Build history of the part. All positions in model axes, mm. Round coordinates to 2 decimals unless told otherwise and drop trailing zeros. Loops run counter-clockwise (first coordinate to the right, second up) from the corner with the lowest first, then second, coordinate; pieces in that order, holes last. Notation, with made-up numbers: (22, 79.5) - (56, 79.5) arc R25 cw to (56, 112.5) - close; hole circle Ø1 at (-34, 85.25). An arc over 180 degrees is marked (long way). Put each result on its own line as item: value. Start each with the question number.
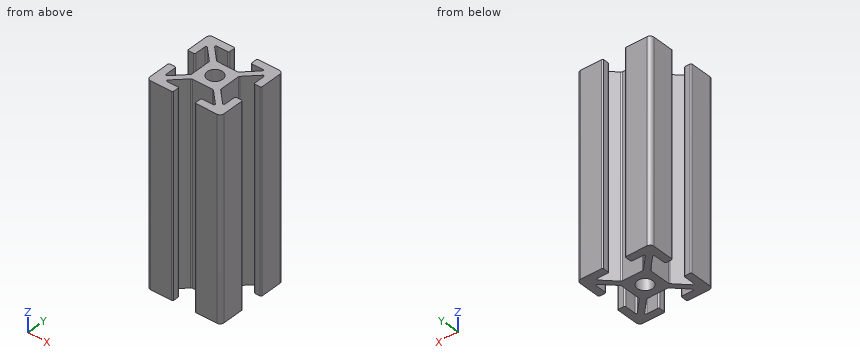
Autodesk Inventor part; units mm, degrees
ref_plane "YZ Plane" through (0, 0, 0) normal (1, 0, 0) x (0, 1, 0)
ref_plane "XZ Plane" through (0, 0, 0) normal (0, 1, 0) x (-1, 0, 0)
ref_plane "XY Plane" through (0, 0, 0) normal (0, 0, 1) x (1, 0, 0)
sketch "Skizze1" plane through (0, 0, 0) normal (0, 0, 1) x (1, 0, 0)
  line L0 (-20.0059, 0) -> (20.0059, 0)
  line L1 (0, -20.0059) -> (0, 20.0059)
  line L2 (-14.2899, 0) -> (14.2899, 0)
  line L3 (0, -14.2899) -> (0, 14.2899)
  line L4 (-10, -10) -> (10, 10) construction
  line L5 (10, -10) -> (-10, 10) construction
  line L6 (-8, -8) -> (8, 8) construction
  line L7 (8, -8) -> (-8, 8) construction
  line L8 (-2.7322, -4) -> (2.7322, -4)
  line L9 (4, -2.7322) -> (4, 2.7322)
  line L10 (2.7322, 4) -> (-2.7322, 4)
  line L11 (-4, 2.7322) -> (-4, -2.7322)
  line L12 (-4, -4) -> (4, 4) construction
  line L13 (4, -4) -> (-4, 4) construction
  arc A0 (-9, 10) -> (-10, 9) centre (-9, 9) ccw
  arc A1 (10, 9) -> (9, 10) centre (9, 9) ccw
  arc A2 (9, -10) -> (10, -9) centre (9, -9) ccw
  arc A3 (-10, -9) -> (-9, -10) centre (-9, -9) ccw
  line L14 (-3, 9.7) -> (-3, 8.3)
  line L15 (3, 9.7) -> (3, 8.3)
  line L16 (6.2151, 8) -> (3.3, 8)
  line L17 (-3.3, 8) -> (-6.2151, 8)
  line L18 (9, 10) -> (3.3, 10)
  line L19 (-3.3, 10) -> (-9, 10)
  line L20 (-9.7, -3) -> (-8.3, -3)
  line L21 (-9.7, 3) -> (-8.3, 3)
  line L22 (-8, 6.2151) -> (-8, 3.3)
  line L23 (-8, -3.3) -> (-8, -6.2151)
  line L24 (-10, 9) -> (-10, 3.3)
  line L25 (-10, -3.3) -> (-10, -9)
  line L26 (-3, -8.3) -> (-3, -9.7)
  line L27 (3, -8.3) -> (3, -9.7)
  line L28 (-9, -10) -> (-3.3, -10)
  line L29 (3.3, -10) -> (9, -10)
  line L30 (-6.2151, -8) -> (-3.3, -8)
  line L31 (3.3, -8) -> (6.2151, -8)
  line L32 (8.3, 3) -> (9.7, 3)
  line L33 (8.3, -3) -> (9.7, -3)
  line L34 (8, -6.2151) -> (8, -3.3)
  line L35 (8, 3.3) -> (8, 6.2151)
  line L36 (10, -9) -> (10, -3.3)
  line L37 (10, 3.3) -> (10, 9)
  arc A4 (-10, 3.3) -> (-9.7, 3) centre (-9.7, 3.3) ccw
  arc A5 (-8.3, 3) -> (-8, 3.3) centre (-8.3, 3.3) ccw
  arc A6 (-9.7, -3) -> (-10, -3.3) centre (-9.7, -3.3) ccw
  arc A7 (-8, -3.3) -> (-8.3, -3) centre (-8.3, -3.3) ccw
  arc A8 (-3.3, -10) -> (-3, -9.7) centre (-3.3, -9.7) ccw
  arc A9 (-3, -8.3) -> (-3.3, -8) centre (-3.3, -8.3) ccw
  arc A10 (3, -9.7) -> (3.3, -10) centre (3.3, -9.7) ccw
  arc A11 (3.3, -8) -> (3, -8.3) centre (3.3, -8.3) ccw
  arc A12 (8.3, -3) -> (8, -3.3) centre (8.3, -3.3) ccw
  arc A13 (10, -3.3) -> (9.7, -3) centre (9.7, -3.3) ccw
  arc A14 (8, 3.3) -> (8.3, 3) centre (8.3, 3.3) ccw
  arc A15 (9.7, 3) -> (10, 3.3) centre (9.7, 3.3) ccw
  arc A16 (3, 8.3) -> (3.3, 8) centre (3.3, 8.3) ccw
  arc A17 (3.3, 10) -> (3, 9.7) centre (3.3, 9.7) ccw
  arc A18 (-3.3, 8) -> (-3, 8.3) centre (-3.3, 8.3) ccw
  arc A19 (-3, 9.7) -> (-3.3, 10) centre (-3.3, 9.7) ccw
  line L38 (-7.4879, 6.4272) -> (-4.1464, 3.0858)
  line L39 (-6.4272, 7.4879) -> (-3.0858, 4.1464)
  line L40 (-6.4272, -7.4879) -> (-3.0858, -4.1464)
  line L41 (-7.4879, -6.4272) -> (-4.1464, -3.0858)
  arc A20 (-7.4879, 6.4272) -> (-8, 6.2151) centre (-7.7, 6.2151) ccw
  arc A21 (-6.2151, 8) -> (-6.4272, 7.4879) centre (-6.2151, 7.7) ccw
  arc A22 (-8, -6.2151) -> (-7.4879, -6.4272) centre (-7.7, -6.2151) ccw
  arc A23 (-6.4272, -7.4879) -> (-6.2151, -8) centre (-6.2151, -7.7) ccw
  line L42 (6.4272, -7.4879) -> (3.0858, -4.1464)
  line L43 (4.1464, -3.0858) -> (7.4879, -6.4272)
  arc A24 (6.2151, -8) -> (6.4272, -7.4879) centre (6.2151, -7.7) ccw
  arc A25 (7.4879, -6.4272) -> (8, -6.2151) centre (7.7, -6.2151) ccw
  line L44 (4.1464, 3.0858) -> (7.4879, 6.4272)
  line L45 (3.0858, 4.1464) -> (6.4272, 7.4879)
  arc A26 (6.4272, 7.4879) -> (6.2151, 8) centre (6.2151, 7.7) ccw
  arc A27 (8, 6.2151) -> (7.4879, 6.4272) centre (7.7, 6.2151) ccw
  arc A28 (-3.0858, 4.1464) -> (-2.7322, 4) centre (-2.7322, 4.5) ccw
  arc A29 (-4, 2.7322) -> (-4.1464, 3.0858) centre (-4.5, 2.7322) ccw
  arc A30 (2.7322, 4) -> (3.0858, 4.1464) centre (2.7322, 4.5) ccw
  arc A31 (4.1464, 3.0858) -> (4, 2.7322) centre (4.5, 2.7322) ccw
  arc A32 (-4.1464, -3.0858) -> (-4, -2.7322) centre (-4.5, -2.7322) ccw
  arc A33 (-2.7322, -4) -> (-3.0858, -4.1464) centre (-2.7322, -4.5) ccw
  arc A34 (3.0858, -4.1464) -> (2.7322, -4) centre (2.7322, -4.5) ccw
  arc A35 (4, -2.7322) -> (4.1464, -3.0858) centre (4.5, -2.7322) ccw
  circle A36 centre (0, 0) radius 2.1
  point P0 (3, 8.9014)
  point P1 (-3, 9.1415)
  point P2 (-8.9764, -3)
  point P3 (-9.1265, 3)
  point P4 (3, -9.1251)
  point P5 (-3, -9.1251)
  point P6 (9.1101, -3)
  point P7 (9.1101, 3)
  dimension "d0" = 20
  dimension "d1" = 20
  dimension "d2" = 16
  dimension "d3" = 16
  dimension "d4" = 8
  dimension "d5" = 8
  dimension "d6" = 1
  dimension "d7" = 6
  dimension "d8" = 6
  dimension "d9" = 6
  dimension "d10" = 6
  dimension "d11" = 0.3
  dimension "d12" = 1.5
  dimension "d13" = 1.5
  dimension "d14" = 0.3
  dimension "d15" = 1.5
  dimension "d16" = 0.3
  dimension "d17" = 1.5
  dimension "d18" = 0.3
  dimension "d19" = 0.5
  dimension "d20" = 4.2
  dimension "d21" = 45
  dimension "d22" = 10
  dimension "d23" = 10
  dimension "d24" = 4
  dimension "d25" = 4
  dimension "d26" = 10
  dimension "d27" = 8
  dimension "d28" = 4
  dimension "d29" = 4
  dimension "d30" = 10
  dimension "d31" = 9.1101
  dimension "d32" = 8
  dimension "d33" = 4
  dimension "d34" = 8.9014
  dimension "d35" = 9.1251
  dimension "d36" = 9.1415
  dimension "d37" = 8.9764
  dimension "d38" = 9.1265
extrude "Extrusion1" add sketch "Skizze1" against normal blind 54 contours L11 A29 L38 A20 L22 A5 L21 A4 L24 A0 L19 A19 L14 A18 L17 A21 L39 A28 L10 L1 A36 L0 | L0 A36 L1 L8 A33 L40 A23 L30 A9 L26 A8 L28 A3 L25 A6 L20 A7 L23 A22 L41 A32 L11 | L1 L10 A30 L45 A26 L16 A16 L15 A17 L18 A1 L37 A15 L32 A14 L35 A27 L44 A31 L9 L0 A36 | A36 L0 L9 A35 L43 A25 L34 A12 L33 A13 L36 A2 L29 A10 L27 A11 L31 A24 L42 A34 L8 L1
properties part number "I Strebe Motorhalterung waagecht" material "Aluminium 6061"
1) Slice it at A-A, the plane y = 0. Write the cut outline in (x, z).
2) Drill centre lines: line 1 (Y direction, x = 8.75, z = -36.5); line 2 (Y direction, x = 0, z = -36.5); line 3 (X direction, y = 3.5, z = -21.5). Where is each one in solid material? Low to high. Write a range as [from, to].
3) Drop flat-ended pins along their axis: pin 1 Ø1 at (x, z) = (-2, -37.5) entering from +Y; pin 2 Ø4.5 at (y, z) = (-1, -30) entering from +X; pin 3 Ø4 at (x, y) = (0, 7) entering from +Z; pin 4 Ø2.5 at (y, z) = (0, -29) entering from -X. Give the stop position or say it passes through.
4) Slice it at C-C, the plane y = 5.5. Write the cut outline in (x, z), and give its area (3 significant figures).
Taken from the geometry:
1. outline: (-4, -54) - (-2.1, -54) - (-2.1, 0) - (-4, 0) - close; (2.1, -54) - (4, -54) - (4, 0) - (2.1, 0) - close
2. line 1: y = [-10, -3], [3, 10]
2. line 2: y = [-4, -2.1], [2.1, 4]
2. line 3: x = [-10, -8], [-4.56, 4.56], [8, 10]
3. pin 1: stops at y = 4
3. pin 2: stops at x = 10
3. pin 3: passes through
3. pin 4: stops at x = -4
4. outline: (-10, -54) - (-8, -54) - (-8, 0) - (-10, 0) - close; (-6.56, -54) - (-4.44, -54) - (-4.44, 0) - (-6.56, 0) - close; (4.44, -54) - (6.56, -54) - (6.56, 0) - (4.44, 0) - close; (8, -54) - (10, -54) - (10, 0) - (8, 0) - close
4. area: 445 mm2
